For this review, take the finished solid that the model builds, in its own axes (mm). Face numbers are marked on the shaded views. A direction names the side the tool comes from. Give positions to 0.01 mm unless a question says otherwise; leave off trailing zeros. Write each loop counter-clockwise with the first axis right and the second up, starting at its lowest first coordinate (ties: lowest second). Pieces come first, ordered by that corner, then holes.
1) Machinability: for the marked faces 5 and 6, which of the approach directions +Z, -Z, +X, -X, +Y, -Y give a long, thin tool a straight path to every point of the face, cutting with its end or side? Answer none if there is none.
2) We need section A-A on z = -55. Give the boundary of the cut face in (x, y).
3) Draft analysis for pull direction X (two halves, no side actions). For the marked faces 1, 2, 3 and 4, state which applies: pulls with the +X half, pulls with the -X half, needs draft (parallel to the pull), parting line crosses it, or undercut.
4) For P1, Ø1, axis at x = -49.5, z = -18, coming from the +Y side, flat-tipped, find the tip position at first contact; note if it passes through.
5) We need section C-C on x = -62. Give the boundary of the cut face in (y, z).
6) We need section B-B on y = 94. Give the boundary of the cut face in (x, z), and give its area (3 significant figures).
7) Wall thickness on line 1 along X through (y, z) = (71.5, -70.5); line 2 along Z through (x, y) = (-68, 33); line 3 along Y through (x, z) = (-26.5, -11.5): over which ranges is each line inside the solid? List them lowest first.
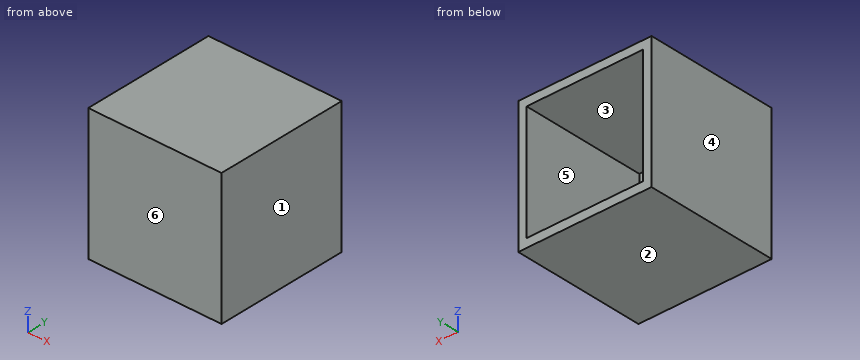
Autodesk Inventor part; units mm, degrees
ref_plane "YZ Plane" through (0, 0, 0) normal (1, 0, 0) x (0, 1, 0)
ref_plane "XZ Plane" through (0, 0, 0) normal (0, 1, 0) x (-1, 0, 0)
ref_plane "XY Plane" through (0, 0, 0) normal (0, 0, 1) x (1, 0, 0)
sketch "Sketch1" plane through (0, 0, 0) normal (0, 1, 0) x (-1, 0, 0)
  line L0 (0, 0) -> (101.6, 0)
  line L1 (101.6, 0) -> (101.6, -101.6)
  line L2 (101.6, -101.6) -> (0, -101.6)
  line L3 (0, -101.6) -> (0, 0)
  dimension "d0" = 101.6
  dimension "d1" = 101.6
extrude "Extrusion1" add sketch "Sketch1" along normal blind 6.35
sketch "Sketch2" plane through (0, 6.35, 0) normal (0, 1, 0) x (1, 0, 0)
  line L0 (0, 0) -> (0, 6.35)
  line L1 (0, 0) -> (0, 101.6)
  line L2 (-6.35, 6.35) -> (-95.25, 6.35)
  line L3 (0, 0) -> (-101.6, 0)
  line L4 (-101.6, 0) -> (0, 0)
  line L5 (-101.6, 0) -> (-101.6, 101.6)
  line L6 (-101.6, 101.6) -> (0, 101.6)
  line L7 (0, 0) -> (0, 101.6)
  line L8 (-101.6, 0) -> (-95.25, 0)
  line L9 (-95.25, 6.35) -> (-95.25, 94.9949)
  line L10 (-95.25, 94.9949) -> (-6.35, 94.9949)
  line L11 (-6.35, 6.35) -> (-6.35, 94.9949)
extrude "Extrusion2" add sketch "Sketch2" along normal blind 95.25
properties part number "gear box"
Results list:
1. face 5: +Y
1. face 6: +Z, -Z, +X, -X, -Y
2. outline: (-101.6, 0) - (0, 0) - (0, 101.6) - (-6.35, 101.6) - (-6.35, 6.35) - (-95.25, 6.35) - (-95.25, 101.6) - (-101.6, 101.6) - close
3. face 1: pulls with the +X half
3. face 2: needs draft
3. face 3: undercut
3. face 4: pulls with the -X half
4. P1: stops at y = 6.35
5. outline: (0, -101.6) - (101.6, -101.6) - (101.6, -94.99) - (6.35, -94.99) - (6.35, -6.35) - (101.6, -6.35) - (101.6, 0) - (0, 0) - close
6. outline: (-101.6, -101.6) - (0, -101.6) - (0, 0) - (-101.6, 0) - close; hole (-95.25, -94.99) - (-6.35, -94.99) - (-6.35, -6.35) - (-95.25, -6.35) - close
6. area: 2,440 mm2
7. line 1: x = -101.6 to -95.25, -6.35 to 0
7. line 2: z = -101.6 to -94.99, -6.35 to 0
7. line 3: y = 0 to 6.35
